```python
from build123d import *

# Parameters (mm, degrees)
BOSS_EXTRUDE1_DEPTH = 10


with BuildPart() as part:
    # Sketch1 → Boss-Extrude1 (new body)
    with BuildSketch(Plane.XY):
        with BuildLine():
            Line((215.829586762, -10.16), (383.521789204, -10.16))
            ThreePointArc((383.521789204, -10.16), (437.403325931, -32.478463274), (459.721789204, -86.36))
            Line((459.721789204, -86.36), (459.721789204, -469.9))
            Line((459.721789204, -469.9), (408.921789204, -469.9))
            Line((408.921789204, -469.9), (408.921789204, -459.74))
            Line((408.921789204, -459.74), (332.721789204, -459.74))
            Line((332.721789204, -459.74), (332.721789204, -469.9))
            Line((332.721789204, -469.9), (215.829586762, -469.9))
            Line((215.829586762, -469.9), (215.829586762, -286.36))
            Line((215.829586762, -286.36), (205.663096361, -286.36))
            Line((205.663096361, -286.36), (205.663096361, -210.16))
            Line((205.663096361, -210.16), (215.829586762, -210.16))
            Line((215.829586762, -210.16), (215.829586762, -10.16))
        make_face()
    extrude(amount=-BOSS_EXTRUDE1_DEPTH)


solid = part.part
```
Geometry: final body of the model. Coordinates: model frame, mm. A direction names the side the tool comes from. Round coordinates to 2 decimals unless told otherwise and drop trailing zeros. Order: outer loops, then holes, each group sorted by start corner. A loop starts at its lowest first (then second) coordinate and runs counter-clockwise, first axis right, second up. Notation, with made-up numbers: M 47.5,-29.75 L 59.5,-29.75 A27 cw 59.5,-10.75 Z; hole C 78,60 d2. An arc over 180 degrees is marked long. One line per item, written item: value.
(1) Reachability of faces 1 (the flat face through (211, -286.36, -5)), 2 (the flat face through (332.722, -465, -5)), 3 (the flat face through (211, -210.16, -5)) from +Z, -Z, +X, -X, +Y, -Y: full face, straight path, thin tool, end or side. Return the list, or none.
Result sheet:
face 1: +Z, -Z, -X, -Y
face 2: +Z, -Z, -Y
face 3: +Z, -Z, -X, +Y
(2) Cut plane C-C (x = 444). Return the cut outline in (y, z).
Result sheet:
outline: M -469.9,-10 L -40,-10 L -40,0 L -469.9,0 Z
(3) Pin query (flat end, axial travel): P1, Ø5, axis at y = -125.5, z = -6, coming from the -X side; P2, Ø5, axis at x = 210, z = -7, coming from the +Y side. Return the tip coordinate at first contact, or that it passes through.
Result sheet:
P1: x = 215.83
P2: y = -210.16
(4) Line query: probe 1 along Y at (x, z) = (375.5, -1); probe 2 along X at (y, z) = (-449, -6); probe 3 along Y at (x, z) = (440, -7.5). Output: solid intervals per line, ascending. Write a range as [from, to].
Result sheet:
probe 1: [-459.74, -10.16]
probe 2: [215.83, 459.72]
probe 3: [-469.9, -35.21]
(5) Pull-direction query (X, two-part tool) for faces 4 (the flat face through (215.83, -379, -5)), 5 (the flat face through (334, -237, -10)), 6 (the flat face through (371, -459.74, -5)); classes: pulls with the +X half, pulls with the -X half, needs draft (parallel to the pull), parting line crosses it, or undercut.
Result sheet:
face 4: pulls with the -X half
face 5: needs draft
face 6: undercut
(6) Cut plane A-A (z = -4.5). Return the cut outline in (x, y), and give its area (3 significant figures).
Result sheet:
outline: M 205.66,-286.36 L 215.83,-286.36 L 215.83,-469.9 L 332.72,-469.9 L 332.72,-459.74 L 408.92,-459.74 L 408.92,-469.9 L 459.72,-469.9 L 459.72,-86.36 A76.2 ccw 383.52,-10.16 L 215.83,-10.16 L 215.83,-210.16 L 205.66,-210.16 Z
area: 111,000 mm2
(7) Cut plane B-B (y = -109). Return the cut outline in (x, z).
Result sheet:
outline: M 215.83,-10 L 459.72,-10 L 459.72,0 L 215.83,0 Z
